```python
from build123d import *

# Parameters (mm, degrees)
F4_DEPTH = 31.75
F6_DEPTH = 3.407345
F7_R     = 5.08


with BuildPart() as f4:
    # F3 (on face) → F4 (new body)
    with BuildSketch(Plane.XZ):
        Polygon((279.374593, 0), (279.374593, 3.406345), (190.476477, 2.827581), (190.476477, 0), align=None)
    extrude(amount=F4_DEPTH)

    # F5 (on face) → F6 (cut, through all)
    with BuildSketch(Plane(origin=(0, 0, 0), x_dir=(1, 0, 0), z_dir=(0, 0, -1))):
        with BuildLine():
            Line((269.849593, 25.4), (200.001477, 25.4))
            ThreePointArc((200.001477, 25.4), (197.756413, 24.470064), (196.826477, 22.225))
            Line((196.826477, 22.225), (196.826477, 9.525))
            ThreePointArc((196.826477, 9.525), (197.756413, 7.279936), (200.001477, 6.35))
            Line((200.001477, 6.35), (269.849593, 6.35))
            ThreePointArc((269.849593, 6.35), (272.094658, 7.279936), (273.024593, 9.525))
            Line((273.024593, 9.525), (273.024593, 22.225))
            ThreePointArc((273.024593, 22.225), (272.094658, 24.470064), (269.849593, 25.4))
        make_face()
    extrude(amount=-F6_DEPTH, mode=Mode.SUBTRACT)

    # F7
    f7_edges = [f4.edges().sort_by_distance(p)[0] for p in [
        (279.374593, -31.75, 1.703173),
        (190.476477, -31.75, 1.413791),
        (190.476477, 0, 1.413791),
        (279.374593, 0, 1.703173),
    ]]
    fillet(f7_edges, radius=F7_R)


solid = f4.part
```
CAD build for the part. Positions are in the model's coordinates, mm. A direction names the side the tool comes from. Coordinates: 2 decimals unless noted, no trailing zeros. Write each loop counter-clockwise with the first axis right and the second up, starting at its lowest first coordinate (ties: lowest second). Pieces come first, ordered by that corner, then holes. Notation, with made-up numbers: (66, -33) -> (80, -33) arc R25 ccw to (80, -21) -> close; hole circle Ø4 at (-1.5, 54). An arc over 180 degrees is marked (long way). Return JSON: item names as keys, results as strings. Group by question number.
Q1. Pull direction X, two halves, no side cores. Call faces 1 (the face through (234, -31.75, 2)), 2 (the face through (279.375, -16, 2)), 3 (the face through (196.826, -16, 1)): released by +X, released by -X, zero draft, split by the parting line, or undercut.
Q2. Cut at B-B, the plane y = -11.5. Give the cut face in (x, z) (3 decimals), then the cut area to 3 significant figures.
Q3. Drill centre lines: line 1 (Y direction, x = 269.5, z = 0.2); line 2 (X direction, y = -20.5, z = 0.2); line 3 (Z direction, x = 269, y = -29.5). Where is each one in solid material? Low to high.
Q4. Cut at C-C, the plane x = 253. Give the cut face in (y, z), then the cut area to 3 significant figures.
Q5. Flat gauge pin, fed straight in: pin 1 (8 mm diameter, centred on x = 209, y = -7.5, fed in from +Z). Where does the tip first touch, or does it go through?
Q6. Cut at A-A, the plane z = 1.45. Give the cut face in (x, y) (3 decimals), then the cut area to 3 significant figures.
Q7. Which spindle directions (+Z, -Z, +X, -X, +Y, -Y) get a long thin tool onto all of the face, cutting with end or side? Do faces 4 (the face through (197.732, -7.305, 1.425)), 5 (the face through (277.93, -30.22, 1.73)). Say none if no direction does.
Returned:
{
 "1": {"face 1": "zero draft", "face 2": "released by +X", "face 3": "undercut"},
 "2": {"outline": "(190.476, 0) -> (196.826, 0) -> (196.826, 2.869) -> (190.476, 2.828) -> close; (273.025, 0) -> (279.375, 0) -> (279.375, 3.406) -> (273.025, 3.365) -> close", "area": "39.6 mm2"},
 "3": {"line 1": "y = -31.75 to -25.4, -6.35 to 0", "line 2": "x = 190.48 to 196.83, 273.02 to 279.37", "line 3": "z = 0 to 3.34"},
 "4": {"outline": "(-31.75, 0) -> (-25.4, 0) -> (-25.4, 3.23) -> (-31.75, 3.23) -> close; (-6.35, 0) -> (0, 0) -> (0, 3.23) -> (-6.35, 3.23) -> close", "area": "41.1 mm2"},
 "5": {"pin 1": "stops at z = 2.97"},
 "6": {"outline": "(190.476, -26.67) arc R5.08 ccw to (195.556, -31.75) -> (274.295, -31.75) arc R5.08 ccw to (279.375, -26.67) -> (279.375, -5.08) arc R5.08 ccw to (274.295, 0) -> (195.556, 0) arc R5.08 ccw to (190.476, -5.08) -> close; hole (196.826, -22.225) arc R3.175 ccw to (200.001, -25.4) -> (269.85, -25.4) arc R3.175 ccw to (273.025, -22.225) -> (273.025, -9.525) arc R3.175 ccw to (269.85, -6.35) -> (200.001, -6.35) arc R3.175 ccw to (196.826, -9.525) -> close", "area": "1,360 mm2"},
 "7": {"face 4": "+Z, -Z", "face 5": "+Z, -Z, +X, -Y"}
}
